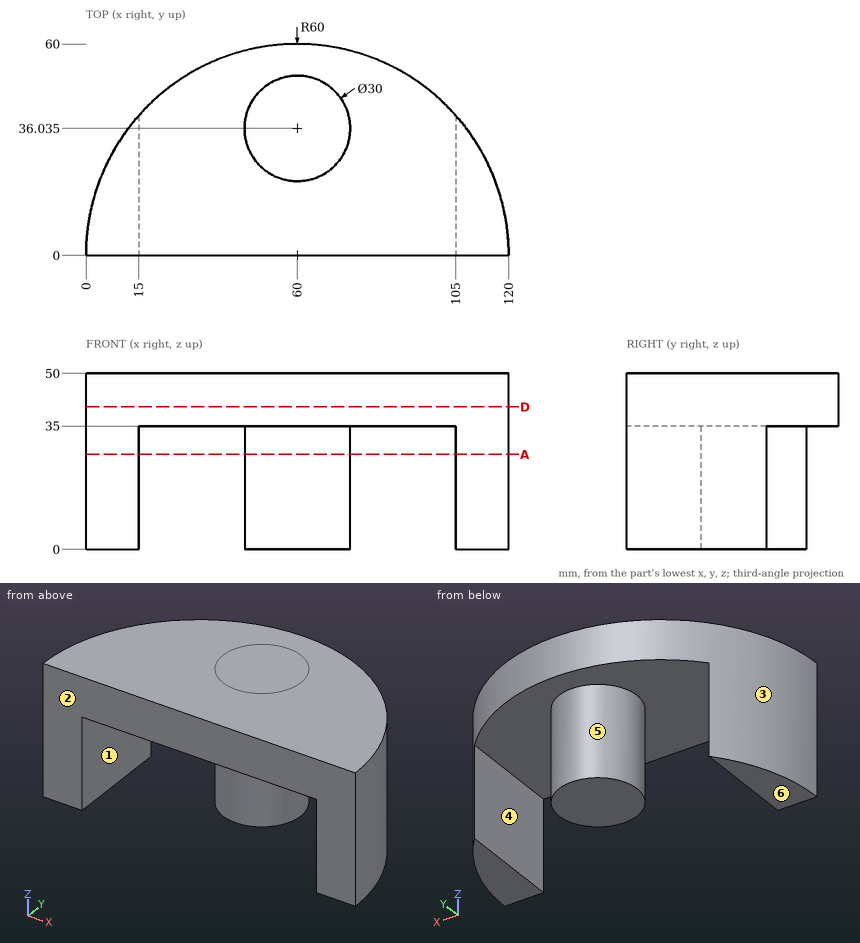
Study the drawing (mm; zero at the part's minimum x, y, z) and answer. A direction names the side the tool comes from. Coordinates: 2 decimals unless noted, no trailing zeros. Write each loop counter-clockwise with the first axis right and the second up, starting at its lowest first coordinate (ties: lowest second). Pieces come first, ordered by that corner, then holes. Notation, with made-up numbers: M 58,-14.75 L 68,-14.75 A7 cw 68,-10.75 Z; hole C -25.75,42.25 d11. An arc over 180 degrees is marked long. Use a Markdown table: item, result. Add a question column.
1. For a pull along X with two mould halves and no side action, classify the marked faces 1, 2 and 3 as +X half, -X half, draft (parallel to the pull), parting line (faces both ways), or undercut.
2. Which of the six approach directions +Z, -Z, +X, -X, +Y, -Y give full straight-line access (tool end or side, diameter ignored) to the marked faces 4, 5 and 6?
3. Section A-A (z = 27) is taken. Give the vertices of the cut face in (x, y) (1 decimal).
4. Section D-D (z = 40.5) is taken. Give the vertices of the cut face in (x, y).
5. Straight lines are drawn through the part: line 1 along X through (y, z) = (26, 24.5) (1 decimal); line 2 along Z through (x, y) = (41, 14); line 3 along X through (y, z) = (38, 6). For each, find the intervals that lie inside material, in ascending order. Write a range as [from, to].
6. Given P1, Ø10.5, axis at y = 27, z = 15.5, coming from the -X side; P2, Ø10, axis at y = 6, z = 40.5, coming from the -X side; P3, Ø4, axis at x = 52.5, z = 23.5, coming from the +Y side, each flat-ended and moving along its own axis, determine where each tip first touches the part or whether it passes through.
Data:
| question | item | result |
|---|---|---|
| 1 | face 1 | undercut |
| 1 | face 2 | draft |
| 1 | face 3 | parting line |
| 2 | face 4 | -Z, +Y, -Y |
| 2 | face 5 | -Z |
| 2 | face 6 | -Z, +X, -X, +Y, -Y |
| 3 | outline | M 0,0 L 15,0 L 15,39.7 A60 ccw Z; C 60,36 d30; M 105,0 L 120,0 A60 ccw 105,39.7 Z |
| 4 | outline | M 0,0 L 120,0 A60 ccw Z |
| 5 | line 1 | x = [5.9, 15], [48.9, 71.1], [105, 114.1] |
| 5 | line 2 | z = [35, 50] |
| 5 | line 3 | x = [13.57, 15], [45.13, 74.87], [105, 106.43] |
| 6 | P1 | stops at x = 4.08 |
| 6 | P2 | stops at x = 0.01 |
| 6 | P3 | stops at y = 49.99 |
